```python
from build123d import *

# Parameters (mm, degrees)
SKETCH1_W           = 300
SKETCH1_H           = 100
BOSS_EXTRUDE1_DEPTH = 3
SKETCH3_W           = 8
SKETCH3_H           = 100
CUT_EXTRUDE2_DEPTH  = 10
SKETCH4_R           = 1.75
CUT_EXTRUDE3_DEPTH  = 4
SKETCH5_R           = 7.5
CUT_EXTRUDE4_DEPTH  = 10
SKETCH6_R           = 1.75
SKETCH6_W           = 9
SKETCH6_H           = 16
CUT_EXTRUDE5_DEPTH  = 10


with BuildPart() as part:
    # Sketch1 → Boss-Extrude1 (new body)
    with BuildSketch(Plane.XY):
        with Locations((150, 50)):
            Rectangle(SKETCH1_W, SKETCH1_H)
    extrude(amount=BOSS_EXTRUDE1_DEPTH)

    # Sketch3 → Cut-Extrude2 (cut)
    with BuildSketch(Plane(origin=(0, 0, 0), x_dir=(-1, 0, 0), z_dir=(0, 0, -1))):
        with Locations((-4, 50)):
            Rectangle(SKETCH3_W, SKETCH3_H)
    extrude(amount=-CUT_EXTRUDE2_DEPTH, mode=Mode.SUBTRACT)

    # Sketch4 → Cut-Extrude3 (cut, through all)
    with BuildSketch(Plane(origin=(0, 0, 0), x_dir=(-1, 0, 0), z_dir=(0, 0, -1))):
        with Locations((-291, 95.5)):
            Circle(SKETCH4_R)
        with Locations((-17, 95.5)):
            Circle(SKETCH4_R)
        with Locations((-17, 7.5)):
            Circle(SKETCH4_R)
        with Locations((-291, 7.5)):
            Circle(SKETCH4_R)
    extrude(amount=-CUT_EXTRUDE3_DEPTH, mode=Mode.SUBTRACT)

    # Sketch5 → Cut-Extrude4 (cut)
    with BuildSketch(Plane(origin=(0, 0, 0), x_dir=(-1, 0, 0), z_dir=(0, 0, -1))):
        with Locations((-48, 60)):
            Circle(SKETCH5_R)
    extrude(amount=-CUT_EXTRUDE4_DEPTH, mode=Mode.SUBTRACT)

    # Sketch6 → Cut-Extrude5 (cut)
    with BuildSketch(Plane(origin=(0, 0, 0), x_dir=(-1, 0, 0), z_dir=(0, 0, -1))):
        with Locations((-275, 45)):
            Circle(SKETCH6_R)
        with Locations((-275, 19)):
            Circle(SKETCH6_R)
        with Locations((-256, 19)):
            Circle(SKETCH6_R)
        with Locations((-256, 45)):
            Circle(SKETCH6_R)
        with Locations((-265.5, 32)):
            Rectangle(SKETCH6_W, SKETCH6_H)
    extrude(amount=-CUT_EXTRUDE5_DEPTH, mode=Mode.SUBTRACT)


solid = part.part
```
Input: part model. Units: mm. Frame: model coordinates. Give positions to 0.01 mm unless a question says otherwise; leave off trailing zeros. Order: outer loops, then holes, each group sorted by start corner. A loop starts at its lowest first (then second) coordinate and runs counter-clockwise, first axis right, second up. Notation, with made-up numbers: (-17, 55) -> (27, 55) arc R24 ccw to (27, 79) -> close; hole circle Ø9 at (80, 26.5). An arc over 180 degrees is marked (long way). Write each question's results on one line, items separated by ' | '. Start each with the question number.
Item 1: Line query: line 1 (Y direction, x = 275, z = 1.5); line 2 (Y direction, x = 17, z = 1.5); line 3 (X direction, y = 95.5, z = 2.1). Output: solid intervals per line, ascending.
Item 2: Mould query, pull axis Y, two halves, no side actions, for faces 1 (the cylindrical face through (43.968, 66.324, 1.479)), 2 (the flat face through (152, 51, 0)). Classes: pulls with the +Y half, pulls with the -Y half, needs draft (parallel to the pull), parting line crosses it, or undercut.
Item 3: Cut plane B-B on y = 28.5. Return the cut outline in (x, z), then the cut area to 3 significant figures.
Item 4: Cut plane A-A on x = 48. Return the cut outline in (y, z), then the cut area to 3 significant figures.
Established:
1) line 1: 0 to 17.25, 20.75 to 43.25, 46.75 to 100 | line 2: 0 to 5.75, 9.25 to 93.75, 97.25 to 100 | line 3: 8 to 15.25, 18.75 to 289.25, 292.75 to 300
2) face 1: undercut | face 2: needs draft
3) outline: (8, 0) -> (261, 0) -> (261, 3) -> (8, 3) -> close; (270, 0) -> (300, 0) -> (300, 3) -> (270, 3) -> close | area: 849 mm^2
4) outline: (0, 0) -> (52.5, 0) -> (52.5, 3) -> (0, 3) -> close; (67.5, 0) -> (100, 0) -> (100, 3) -> (67.5, 3) -> close | area: 255 mm^2
